The model under review builds one solid part; all positions refer to its coordinate system, in mm. Face numbers are marked on the shaded views. A direction names the side the tool comes from. Round coordinates to 2 decimals unless told otherwise and drop trailing zeros. Write each loop counter-clockwise with the first axis right and the second up, starting at its lowest first coordinate (ties: lowest second). Pieces come first, ordered by that corner, then holes. Notation, with made-up numbers: (-13.75, 15) - (-7.75, 15) arc R25 cw to (-7.75, 49) - close; hole circle Ø6 at (-13, 20.5). An arc over 180 degrees is marked (long way). Use one line per item in the form item = value.
from build123d import *

# Parameters (mm, degrees)
CYLINDER001_R     = 4
CYLINDER001_DEPTH = 20
PAD_DEPTH         = 10
CYLINDER_R        = 10
CYLINDER_DEPTH    = 20
CYLINDER005_R     = 8.5
CYLINDER005_DEPTH = 20
CYLINDER004_R     = 8.5
CYLINDER004_DEPTH = 20


with BuildPart() as cylinder001:
    # Cylinder001 → Cylinder001 (new body)
    with BuildSketch(Plane.ZY.offset(-10)):
        Circle(CYLINDER001_R)
    extrude(amount=CYLINDER001_DEPTH)


with BuildPart() as negative_fusion:
    # Sketch → Pad (new body)
    with BuildSketch(Plane.YZ):
        Polygon((6.1, -3.521837), (6.1, 3.521837), (0, 7.043673), (-6.1, 3.521837), (-6.1, -3.521837), (0, -7.043673), align=None)
    extrude(amount=-PAD_DEPTH)


with BuildPart() as negative_fusion_1:
    # Body placement: moved
    add(negative_fusion.part.moved(Location((10, 0, 0))))

    # Fusion: union Cylinder001
    add(cylinder001.part)


with BuildPart() as cylinder:
    # Cylinder → Cylinder (new body)
    with BuildSketch(Plane(origin=(0, -10, 0), x_dir=(1, 0, 0), z_dir=(0, 1, 0))):
        Circle(CYLINDER_R)
    extrude(amount=CYLINDER_DEPTH)


with BuildPart() as cylinder005:
    # Cylinder005 → Cylinder005 (new body)
    with BuildSketch(Plane(origin=(0, 10, 0), x_dir=(-1, 0, 0), z_dir=(0, 1, 0))):
        Circle(CYLINDER005_R)
    extrude(amount=CYLINDER005_DEPTH)


with BuildPart() as cut:
    # Cylinder004 → Cylinder004 (new body)
    with BuildSketch(Plane(origin=(0, -10, 0), x_dir=(-1, 0, 0), z_dir=(0, -1, 0))):
        Circle(CYLINDER004_R)
    extrude(amount=CYLINDER004_DEPTH)

    # Fusion001: union Cylinder, Cylinder005
    add(cylinder.part)
    add(cylinder005.part)

    # Cut: cut Negative Fusion
    add(negative_fusion_1.part, mode=Mode.SUBTRACT)


solid = cut.part
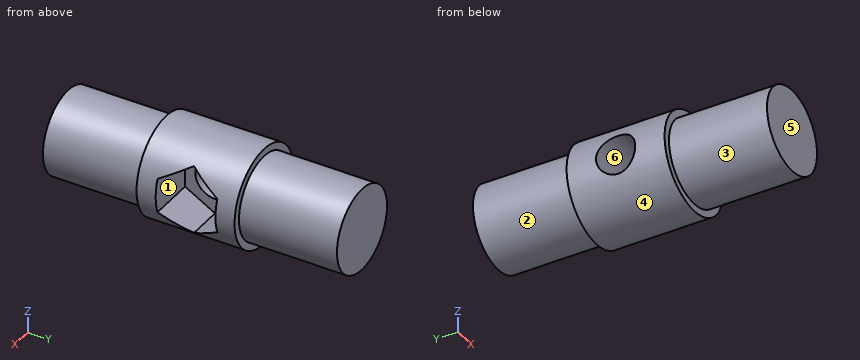
(1) The part is to be moulded in two halves that separate along Z. For the marked faces 4, 5 and 6, say which applies: +Z half, -Z half, draft (parallel to the pull), parting line (faces both ways), or undercut.
Geometry results:
face_4 = parting line
face_5 = draft
face_6 = undercut
(2) To check wall thickness, follow L1, parallel to Y at x = -5.75, z = 0; L2, parallel to Y at x = 6.75, z = -1; L3, parallel to X at y = -25, z = 0. State the ranges of each line that lie inside material, in increasing order.
Geometry results:
L1 = -30 to -4, 4 to 30
L2 = -30 to -6.1, 6.1 to 30
L3 = -8.5 to 8.5
(3) Add section A-A on z = 2.5. Write out the cut boundary in (x, y), then the cut area to 3 significant figures.
Geometry results:
outline = (-9.68, -10) - (-8.12, -10) - (-8.12, -30) - (8.12, -30) - (8.12, -10) - (9.68, -10) - (9.68, -6.1) - (0, -6.1) - (0, -3.12) - (-9.68, -3.12) - close; (-9.68, 3.12) - (0, 3.12) - (0, 6.1) - (9.68, 6.1) - (9.68, 10) - (8.12, 10) - (8.12, 30) - (-8.12, 30) - (-8.12, 10) - (-9.68, 10) - close
area = 859 mm2
(4) Insertion check: P1, Ø6, axis at y = -9.5, z = -6, coming from the -X side; P2, Ø2, axis at x = 7, y = 21.5, coming from the -Z side; P3, Ø6.5, axis at y = 0, z = 0, coming from the -X side; P4, Ø4, axis at y = 2, z = 4, coming from the -X side. Each pin has a flat end and moves straight along its axis. Give the tip position at first contact, or say it passes through.
Geometry results:
P1 = -9.54
P2 = -6.02
P3 = through
P4 = -9.71
(5) Add section B-B on x = 5.25. Write out the cut boundary in (y, z).
Geometry results:
outline = (-30, -6.68) - (-10, -6.68) - (-10, -8.51) - (10, -8.51) - (10, -6.68) - (30, -6.68) - (30, 6.68) - (10, 6.68) - (10, 8.51) - (-10, 8.51) - (-10, 6.68) - (-30, 6.68) - close; hole (-6.1, -3.52) - (0, -7.04) - (6.1, -3.52) - (6.1, 3.52) - (0, 7.04) - (-6.1, 3.52) - close
(6) Machinability: for the marked faces 1, 2 and 3, which of the approach directions +Z, -Z, +X, -X, +Y, -Y give a long, thin tool a straight path to every point of the face, cutting with its end or side? Answer none if there is none.
Geometry results:
face_1 = +X
face_2 = +Y
face_3 = -Y
(7) Add section D-D on y = -15.5. Write out the cut boundary in (x, z), then the cut area to 3 significant figures.
Geometry results:
outline = circle Ø17 at (0, 0)
area = 227 mm2
(8) Add section C-C on z = 0. Write out the cut boundary in (x, y).
Geometry results:
outline = (-10, -10) - (-8.5, -10) - (-8.5, -30) - (8.5, -30) - (8.5, -10) - (10, -10) - (10, -6.1) - (0, -6.1) - (0, -4) - (-10, -4) - close; (-10, 4) - (0, 4) - (0, 6.1) - (10, 6.1) - (10, 10) - (8.5, 10) - (8.5, 30) - (-8.5, 30) - (-8.5, 10) - (-10, 10) - close
